Geometry: final body of the model. Coordinates: model frame, mm. Face numbers are marked on the shaded views. A direction names the side the tool comes from. Give positions to 0.01 mm unless a question says otherwise; leave off trailing zeros. Write each loop counter-clockwise with the first axis right and the second up, starting at its lowest first coordinate (ties: lowest second). Pieces come first, ordered by that corner, then holes.
Q1. Section A-A (z = 2.5). Return the cut outline in (x, y).
Q2. Section B-B (x = 5.5). Return the cut outline in (y, z).
Q3. Reachability of the marked faces 5 and 6 from +Z, -Z, +X, -X, +Y, -Y: full face, straight path, thin tool, end or side. Return the list, or none.
Q4. Line query: line 1 (X direction, y = -1, z = 5.75); line 2 (X direction, y = 0.7, z = 0); line 3 (Z direction, x = -2, y = -0.4). Output: solid intervals per line, ascending.
Q5. Section C-C (y = -0.2). State how many separate pieces and enclosed holes the cut face has, plus the area to 3 significant figures.
Q6. Pin query (flat end, axial travel): pin 1 Ø2 at (x, z) = (-0.98, 8.77) entering from -Y. Return the tip coordinate at first contact, or that it passes through.
Q7. Mould query, pull axis Z, two halves, no side actions, for the marked faces 1, 2, 3 and 4. Classes: +Z half, -Z half, draft (parallel to the pull), parting line (faces both ways), or undercut.
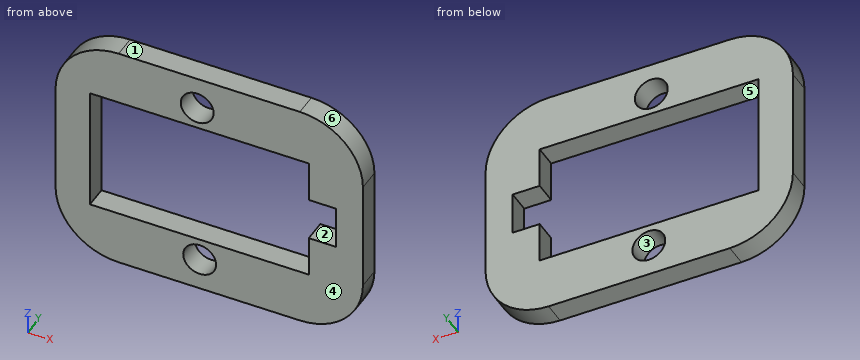
from build123d import *

# Parameters (mm, degrees)
SKETCH2_R           = 1.825
BOSS_EXTRUDE1_DEPTH = 1.25


with BuildPart() as part:
    # Sketch2 → Boss-Extrude1 (new, symmetric)
    with BuildSketch(Plane(origin=(0, 0, 0), x_dir=(1, 0, 0), z_dir=(0, 1, 0))):
        with BuildLine():
            Line((-9.701491638, 14.016578985), (10.422938362, 14.016578985))
            ThreePointArc((10.422938362, 14.016578985), (15.37268583, 11.966326454), (17.422938362, 7.016578985))
            Line((17.422938362, 7.016578985), (17.422938362, -5.461573784))
            ThreePointArc((17.422938362, -5.461573784), (15.37268583, -10.411321253), (10.422938362, -12.461573784))
            Line((10.422938362, -12.461573784), (-9.701491638, -12.461573784))
            ThreePointArc((-9.701491638, -12.461573784), (-14.651239107, -10.411321253), (-16.701491638, -5.461573784))
            Line((-16.701491638, -5.461573784), (-16.701491638, 7.016578985))
            ThreePointArc((-16.701491638, 7.016578985), (-14.651239107, 11.966326454), (-9.701491638, 14.016578985))
        make_face()
        with Locations(Location((-0.702610465, 10.366481865, 0), (0, 0, 270))):
            Circle(SKETCH2_R, mode=Mode.SUBTRACT)
        with Locations(Location((-0.97805, -8.773518135, 0), (0, 0, 270))):
            Circle(SKETCH2_R, mode=Mode.SUBTRACT)
        Polygon((-12.878350873, 7.83354898), (11.411239127, 7.83354898), (11.411239127, 3.2058826), (14.411239127, 3.2058826), (14.411239127, -1.6439074), (11.411239127, -1.6439074), (11.411239127, -6.27157378), (-12.878350873, -6.27157378), align=None, mode=Mode.SUBTRACT)
    extrude(amount=BOSS_EXTRUDE1_DEPTH, both=True)


solid = part.part
Computed:
1. outline: (-16.7, -1.25) - (-12.88, -1.25) - (-12.88, 1.25) - (-16.7, 1.25) - close; (11.41, -1.25) - (17.42, -1.25) - (17.42, 1.25) - (11.41, 1.25) - close
2. outline: (-1.25, -14.02) - (1.25, -14.02) - (1.25, -7.83) - (-1.25, -7.83) - close; (-1.25, 6.27) - (1.25, 6.27) - (1.25, 12.46) - (-1.25, 12.46) - close
3. face 5: +Y, -Y
3. face 6: +Z, +X, +Y, -Y
4. line 1: x = -16.7 to -12.88, 11.41 to 17.42
4. line 2: x = -16.7 to -12.88, 14.41 to 17.42
4. line 3: z = -14.02 to -11.65, -9.08 to -7.83, 6.27 to 7.26, 10.29 to 12.46
5. separate pieces: 1
5. enclosed holes: 3
5. area: 483 mm2
6. pin 1: passes through
7. face 1: +Z half
7. face 2: undercut
7. face 3: undercut
7. face 4: draft
